Job drawing, mm, ordinate dimensions from the low corner. One solid piece. A direction names the side the tool comes from. Round coordinates to 2 decimals unless told otherwise and drop trailing zeros. Write each loop counter-clockwise with the first axis right and the second up, starting at its lowest first coordinate (ties: lowest second). Pieces come first, ordered by that corner, then holes. Notation, with made-up numbers: (47, -8.75) -> (95, -8.75) arc R18 ccw to (95, 21.25) -> close; hole circle Ø11 at (34, 64). An arc over 180 degrees is marked (long way). Use CSV: the item, a comma, the result in double quotes. Start each with the question number.
(1) Probe line 1 (Y direction, x = 12, z = 27.5); line 2 (Y direction, x = 8, z = 19). List the from-to ranges inside material, lowest first. Write a range as [from, to].
(2) Saw through at B-B (z = 44). Give the cut face in (x, y).
(3) Which spindle directions (+Z, -Z, +X, -X, +Y, -Y) get a long thin tool onto all of the face, cutting with end or side? Do the marked faces 1, 2 and 3. Say none if no direction does.
(4) Saw through at C-C (y = 42.5). Give the cut face in (x, z), plus the area to 3 significant figures.
(5) Drop flat-ended pins along their axis: pin 1 (5.5 mm diameter, centred on x = 9, y = 6.5, fed in from +Z); pin 2 (5.5 mm diameter, centred on x = 6.5, y = 31, fed in from +Z); pin 3 (3 mm diameter, centred on x = 3, z = 6, fed in from +Y). Give the stop position or say it passes through.
(6) Saw through at A-A (x = 16.25). Give the cut face in (y, z), plus the area to 3 significant figures.
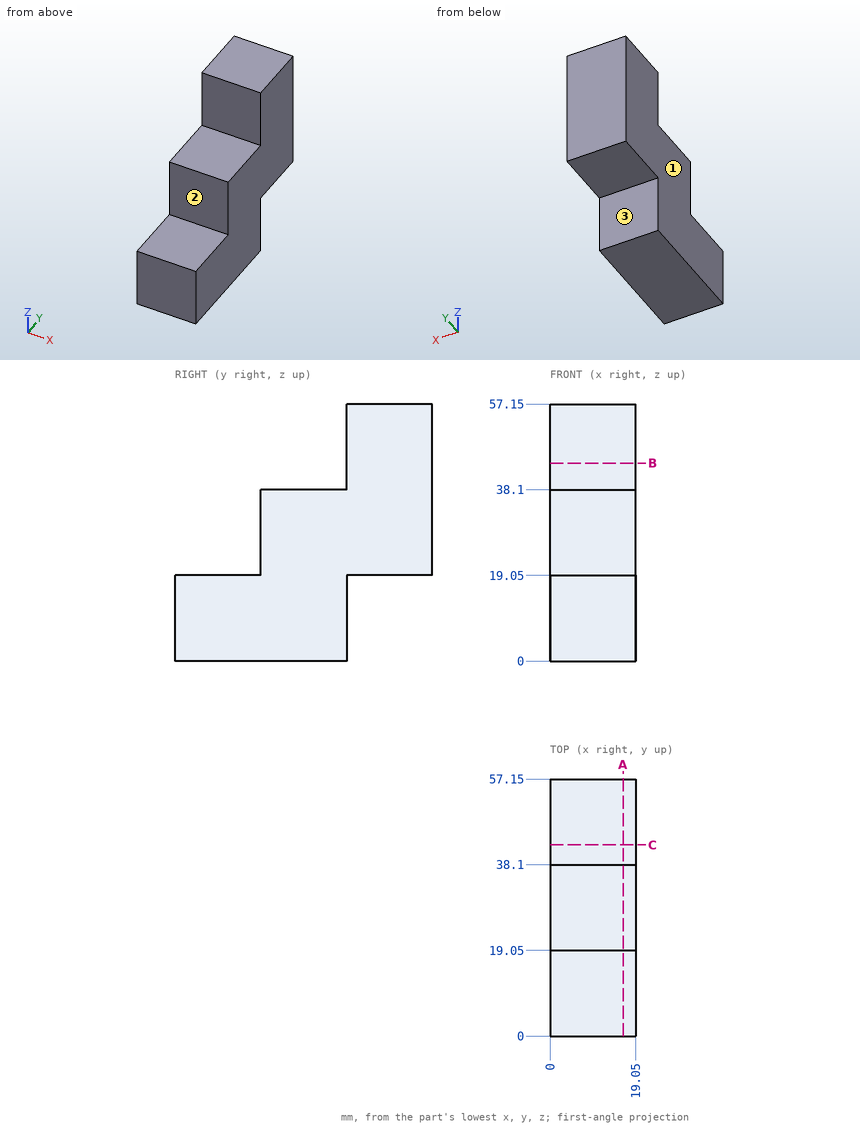
Answers:
1,line 1,"y = [19.05, 57.15]"
1,line 2,"y = [0, 38.1]"
2,outline,"(0, 38.1) -> (19.05, 38.1) -> (19.05, 57.15) -> (0, 57.15) -> close"
3,face 1,"+Z, -Z, -X, +Y, -Y"
3,face 2,"+Z, +X, -X, -Y"
3,face 3,"-Z, +X, -X, +Y"
4,outline,"(0, 19.05) -> (19.05, 19.05) -> (19.05, 57.15) -> (0, 57.15) -> close"
4,area,"726 mm²"
5,pin 1,"stops at z = 19.05"
5,pin 2,"stops at z = 38.1"
5,pin 3,"stops at y = 38.1"
6,outline,"(0, 0) -> (38.1, 0) -> (38.1, 19.05) -> (57.15, 19.05) -> (57.15, 57.15) -> (38.1, 57.15) -> (38.1, 38.1) -> (19.05, 38.1) -> (19.05, 19.05) -> (0, 19.05) -> close"
6,area,"1,810 mm²"
